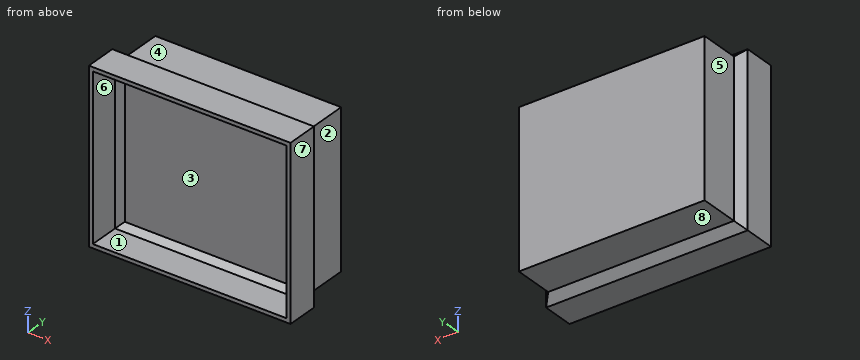
from build123d import *

# Parameters (mm, degrees)
F0_W     = 127.2814720869
F0_H     = 107.5093485415
F1_DEPTH = 25
F2_SIZE  = 5
F3_T     = -2.5
F4_W     = 117.2814720869
F4_H     = 97.5093485415
F5_DEPTH = 25


with BuildPart() as f1:
    # F0 (on Front) → F1 (new body)
    with BuildSketch(Plane.XZ):
        with Locations((-2.2627860308, -9.7043421119)):
            Rectangle(F0_W, F0_H)
    extrude(amount=F1_DEPTH)

    # F2
    f2_edges = [f1.edges().sort_by_distance(p)[0] for p in [
        (61.37795, 0, -9.704342),
        (-2.262786, 0, -63.459016),
        (-65.903522, 0, -9.704342),
        (-2.262786, 0, 44.050332),
    ]]
    chamfer(f2_edges, length=F2_SIZE)

    # F3
    f3_openings = [f1.faces().sort_by_distance(p)[0] for p in [
        (-2.262786, -25, -9.704342),
    ]]
    offset(amount=F3_T, openings=f3_openings)

    # F4 (on face) → F5 (join)
    with BuildSketch(Plane(origin=(0, 0, 0), x_dir=(-1, 0, 0), z_dir=(0, 1, 0))):
        with Locations((2.2627860308, -9.7043421119)):
            Rectangle(F4_W, F4_H)
    extrude(amount=F5_DEPTH)


solid = f1.part
Can you work these out from the model? Positions are in its coordinate system, mm. Face numbers are marked on the shaded views. A direction names the side the tool comes from. Give positions to 0.01 mm unless a question says otherwise; leave off trailing zeros. Order: outer loops, then holes, each group sorted by start corner. A loop starts at its lowest first (then second) coordinate and runs counter-clockwise, first axis right, second up. Notation, with made-up numbers: M 71,-34.5 L 101,-34.5 A15 cw 101,-11.5 Z; hole C 60.5,39.25 d7. An arc over 180 degrees is marked long. One line per item, written item: value.
Item 1: For the marked faces 5, 6, 7 and 8, which set-ups out of +Z, -Z, +X, -X, +Y, -Y let a thin tool reach every point of the face, with its end or its side?
Verdict:
face 5: +Z, -Z, -X, +Y
face 6: -Y
face 7: +Z, -Z, +X, +Y, -Y
face 8: -Z, +X, -X, +Y
Item 2: If we section it at A-A on z = 4.5: Write out the boundary of the cut face in (x, y), and give its area (3 significant figures).
Verdict:
outline: M -65.9,-25 L -63.4,-25 L -63.4,-6.04 L -59.87,-2.5 L 55.34,-2.5 L 58.88,-6.04 L 58.88,-25 L 61.38,-25 L 61.38,-5 L 56.38,0 L 56.38,25 L -60.9,25 L -60.9,0 L -65.9,-5 Z
area: 3,350 mm2
Item 3: If we section it at B-B on y = -12: Write out the boundary of the cut face in (x, z), and give its area (3 significant figures).
Verdict:
outline: M -65.9,-63.46 L 61.38,-63.46 L 61.38,44.05 L -65.9,44.05 Z; hole M -63.4,-60.96 L 58.88,-60.96 L 58.88,41.55 L -63.4,41.55 Z
area: 1,150 mm2
Item 4: If we mould it in two halves opening along X, with no side actions, what happens to the marked faces 1, 2, 3 and 4? For each: pulls with the +X half, pulls with the -X half, needs draft (parallel to the pull), parting line crosses it, or undercut.
Verdict:
face 1: undercut
face 2: pulls with the +X half
face 3: undercut
face 4: needs draft
Item 5: If we section it at C-C on x = -40: Write out the boundary of the cut face in (y, z).
Verdict:
outline: M -25,-63.46 L -5,-63.46 L 0,-58.46 L 25,-58.46 L 25,39.05 L 0,39.05 L -5,44.05 L -25,44.05 L -25,41.55 L -6.04,41.55 L -2.5,38.01 L -2.5,-57.42 L -6.04,-60.96 L -25,-60.96 Z
Item 6: Please list where these lines run through material, in increasing order: line 1 (X direction, y = -12, z = -1.5); line 2 (Z direction, x = -22, y = -16); line 3 (X direction, y = 1.5, z = 29).
Verdict:
line 1: -65.9 to -63.4, 58.88 to 61.38
line 2: -63.46 to -60.96, 41.55 to 44.05
line 3: -60.9 to 56.38
Item 7: For pin 1 (3 mm diameter, centred on y = 8.5, z = 13.5, fed in from +X); pin 2 (6 mm diameter, centred on y = 6.5, z = 23, fed in from -X); pin 3 (7.5 mm diameter, centred on x = -3.5, y = 7.5, fed in from -Z), each with a flat end and sliding along its axis, tell me the tip position at first contact or that it passes through.
Verdict:
pin 1: x = 56.38
pin 2: x = -60.9
pin 3: z = -58.46
Item 8: If we section it at D-D on y = 9: Write out the boundary of the cut face in (x, z).
Verdict:
outline: M -60.9,-58.46 L 56.38,-58.46 L 56.38,39.05 L -60.9,39.05 Z
